```python
from build123d import *

# Parameters (mm, degrees)
CROQUIS1_R              = 85.75
SALIENTE_EXTRUIR1_DEPTH = 105
CROQUIS2_R              = 21
SALIENTE_EXTRUIR2_DEPTH = 10.5
CROQUIS3_R              = 3.5
SALIENTE_EXTRUIR4_DEPTH = 150.5


with BuildPart() as part:
    # Croquis1 → Saliente-Extruir1 (new body)
    with BuildSketch(Plane.XY):
        Circle(CROQUIS1_R)
    extrude(amount=SALIENTE_EXTRUIR1_DEPTH)

    # Croquis2 → Saliente-Extruir2 (add)
    with BuildSketch(Plane.XY):
        Circle(CROQUIS2_R)
    extrude(amount=-SALIENTE_EXTRUIR2_DEPTH)

    # Croquis3 → Saliente-Extruir4 (add)
    with BuildSketch(Plane(origin=(0, 0, 0), x_dir=(-1, 0, 0), z_dir=(0, 0, -1))):
        Circle(CROQUIS3_R)
    extrude(amount=-SALIENTE_EXTRUIR4_DEPTH)


solid = part.part
```
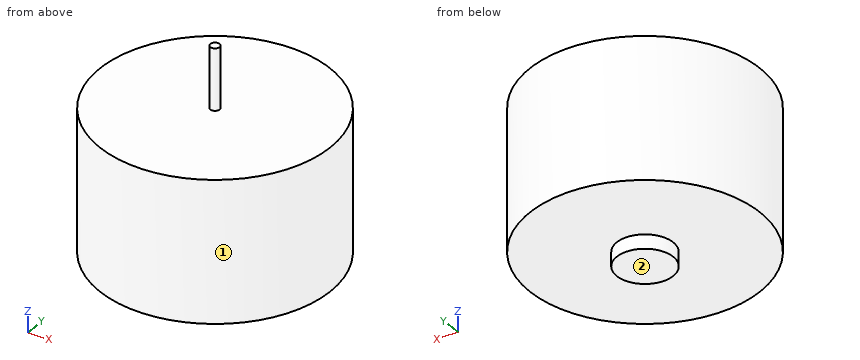
CAD build for the part. Positions are in the model's coordinates, mm. Face numbers are marked on the shaded views. Give positions to 0.01 mm unless a question says otherwise; leave off trailing zeros. Loops run counter-clockwise (first coordinate to the right, second up) from the corner with the lowest first, then second, coordinate; pieces in that order, holes last. Notation, with made-up numbers: (-15, 26) -> (29, 26) arc R12 cw to (29, 31) -> close; hole circle Ø2 at (-15.75, 88). An arc over 180 degrees is marked (long way). Use a Markdown table: item, result.
1. Wall check: L1, parallel to Z at x = 52.5, y = -43.5; L2, parallel to Y at x = 31.5, z = 22; L3, parallel to Y at x = 49, z = 55. Give the ranges that are in metal, low to high. Write a range as [from, to].
Check result:
| item | result |
|---|---|
| L1 | z = [0, 105] |
| L2 | y = [-79.75, 79.75] |
| L3 | y = [-70.37, 70.37] |
2. Flat gauge pins, fed straight in: pin 1 (1.5 mm diameter, centred on y = -26.5, z = 21.5, fed in from -X); pin 2 (2 mm diameter, centred on x = 14.5, z = 59.5, fed in from -Y); pin 3 (1.5 mm diameter, centred on x = -19, z = 81, fed in from -Y). Where does each tip first touch, or does it go through?
Check result:
| item | result |
|---|---|
| pin 1 | stops at x = -81.79 |
| pin 2 | stops at y = -84.68 |
| pin 3 | stops at y = -83.79 |
3. Slice it at C-C (z = 91). List the corners of the cut face in (x, y).
Check result:
| item | result |
|---|---|
| outline | circle Ø171.5 at (0, 0) |
4. Slice it at D-D (x = -26.5). List the corners of the cut face in (y, z).
Check result:
| item | result |
|---|---|
| outline | (-81.55, 0) -> (81.55, 0) -> (81.55, 105) -> (-81.55, 105) -> close |
5. Slice it at A-A (x = 0). List the corners of the cut face in (y, z), plus the area to 3 significant figures.
Check result:
| item | result |
|---|---|
| outline | (-85.75, 0) -> (-21, 0) -> (-21, -10.5) -> (21, -10.5) -> (21, 0) -> (85.75, 0) -> (85.75, 105) -> (3.5, 105) -> (3.5, 150.5) -> (-3.5, 150.5) -> (-3.5, 105) -> (-85.75, 105) -> close |
| area | 18,800 mm^2 |
6. Mould opens along Y. For the marked faces 1 and 2 say: pulls with the +Y half, pulls with the -Y half, needs draft (parallel to the pull), parting line crosses it, or undercut.
Check result:
| item | result |
|---|---|
| face 1 | parting line crosses it |
| face 2 | needs draft |
